Here's the drawing with two shaded views (mm, measured from the low corner). I have some questions. Coordinates: 2 decimals unless noted, no trailing zeros. Loops run counter-clockwise (first coordinate to the right, second up) from the corner with the lowest first, then second, coordinate; pieces in that order, holes last.
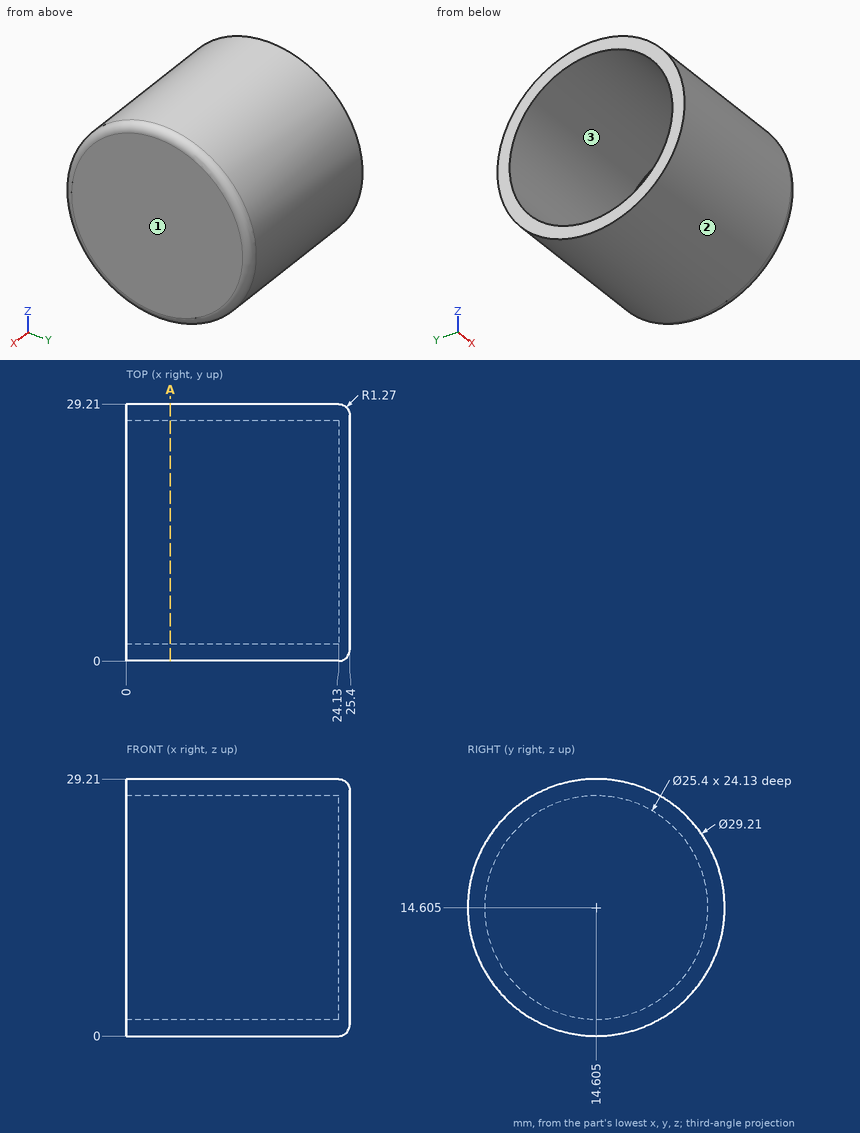
Q1. Please list where these lines run through material, in increasing order: probe 1 along X at (y, z) = (20.5, 18); probe 2 along Z at (x, y) = (12.25, 6.5); probe 3 along Z at (x, y) = (13.25, 13.75).
Q2. We'd pull the mould along Y, two halves only. Please class the marked faces 1, 2 and 3: pulls with the +Y half, pulls with the -Y half, needs draft (parallel to the pull), parting line crosses it, or undercut.
Q3. Suppose I cut it at A-A on x = 5. Write out the boundary of the cut face in (y, z) (3 decimals), and give its area (3 significant figures).
Q4. Will these pins go through, and if not, where does the flat tip stop? P1, Ø5, axis at x = 10, y = 7, coming from the +Z side; P2, Ø10, axis at x = 10.5, y = 4, coming from the -Z side; P3, Ø1, axis at x = 3, y = 7.5, coming from the -Z side.
Check values:
1. probe 1: x = 24.13 to 25.4
1. probe 2: z = 2.46 to 4.83, 24.38 to 26.75
1. probe 3: z = 0.03 to 1.93, 27.28 to 29.18
2. face 1: needs draft
2. face 2: parting line crosses it
2. face 3: undercut
3. outline: circle Ø29.21 at (14.605, 14.605); hole circle Ø25.4 at (14.605, 14.605)
3. area: 163 mm2
4. P1: stops at z = 28.29
4. P2: stops at z = 1.12
4. P3: stops at z = 1.58
